Read the model definition and answer for the solid it produces. Units are mm, in the model's axes. Give positions to 0.01 mm unless a question says otherwise; leave off trailing zeros. Write each loop counter-clockwise with the first axis right and the second up, starting at its lowest first coordinate (ties: lowest second). Pieces come first, ordered by that corner, then holes. Notation, with made-up numbers: (74, 52) -> (105, 52) arc R22 ccw to (105, 73) -> close; hole circle Ø11 at (-34.5, -32). An arc over 180 degrees is marked (long way). Write item = value, one per line.
from build123d import *

# Parameters (mm, degrees)
FILLET1_R          = 0.25
CUT_EXTRUDE1_REACH = 9
SKETCH3_R          = 6


with BuildPart() as part:
    # Sketch2 → Revolve1 (revolve)
    with BuildSketch(Plane.XY):
        with BuildLine():
            Line((0, 0), (7, 0))
            Line((7, 0), (7, 10))
            Line((7, 10), (5.868174923, 9.087607037))
            ThreePointArc((5.868174923, 9.087607037), (3.5, 8.251940939), (1.131825077, 9.087607037))
            Line((1.131825077, 9.087607037), (0, 10))
            Line((0, 10), (0, 0))
        make_face()
    revolve(axis=Axis((0, 0, 0), (1, 0, 0)))

    # Fillet1
    fillet1_edges = [part.edges().sort_by_distance(p)[0] for p in [
        (0, -10, 0),
        (7, -10, 0),
    ]]
    fillet(fillet1_edges, radius=FILLET1_R)

    # Sketch3 → Cut-Extrude1 (cut, up to next)
    with BuildSketch(Plane.ZY, mode=Mode.PRIVATE) as cut_extrude1_sk1:
        Circle(SKETCH3_R)
    cut_extrude1_tool1 = extrude(cut_extrude1_sk1.sketch, amount=-CUT_EXTRUDE1_REACH, mode=Mode.PRIVATE) & part.part
    add(cut_extrude1_tool1.solids().sort_by_distance((0, 0, 0))[0], mode=Mode.SUBTRACT)


solid = part.part
(1) The part is cut by section D-D on x = 1.75. Determine the outline of the cut face in (y, z), plus the area to 3 significant figures.
Checks:
outline = circle Ø17.36 at (0, 0); hole circle Ø12 at (0, 0)
area = 124 mm²
(2) Consider L1, parallel to Z at x = 0.75, y = -3; L2, parallel to Y at x = 4.75, z = 0 (3 decimals); L3, parallel to Y at x = 1.5, z = -5.5. Determine where each line is inside the solid, lowest interval first.
Checks:
L1 = -8.9 to -5.2, 5.2 to 8.9
L2 = -8.465 to -6, 6 to 8.465
L3 = -6.9 to -2.4, 2.4 to 6.9
(3) Given P1, Ø2, axis at x = 3.5, z = 6.5, coming from the -Y side; P2, Ø1, axis at x = 3.5, z = 4.5, coming from the +Y side; P3, Ø1.5, axis at x = 5.5, y = 5.5, coming from the -Z side; P4, Ø1, axis at y = -7.5, z = 0.5, coming from the -X side, each flat-ended and moving along its own axis, determine where each tip first touches the part or whether it passes through.
Checks:
P1 = -6.15
P2 = 7.22
P3 = -7.78
P4 = 0
(4) For a pull along Y with two mould halves and no side action, classify faces 1 (the flat face through (0, -0.1, -6.2)), 2 (the cylindrical face through (3, 0, -6)) as released by +Y, released by -Y, zero draft, split by the parting line, or undercut.
Checks:
face_1 = zero draft
face_2 = undercut
(5) The part is cut by section C-C on x = 3.5. Determine the outline of the cut face in (y, z).
Checks:
outline = circle Ø16.5 at (0, 0); hole circle Ø12 at (0, 0)
(6) The part is cut by section A-A on y = 0. Determine the outline of the cut face in (x, z), plus the area to 3 significant figures.
Checks:
outline = (0, -9.48) arc R0.25 ccw to (0.41, -9.67) -> (1.13, -9.09) arc R3.77 cw to (5.87, -9.09) -> (6.59, -9.67) arc R0.25 ccw to (7, -9.48) -> (7, -6) -> (0, -6) -> close; (0, 6) -> (7, 6) -> (7, 9.48) arc R0.25 ccw to (6.59, 9.67) -> (5.87, 9.09) arc R3.77 cw to (1.13, 9.09) -> (0.41, 9.67) arc R0.25 ccw to (0, 9.48) -> close
area = 39.6 mm²
